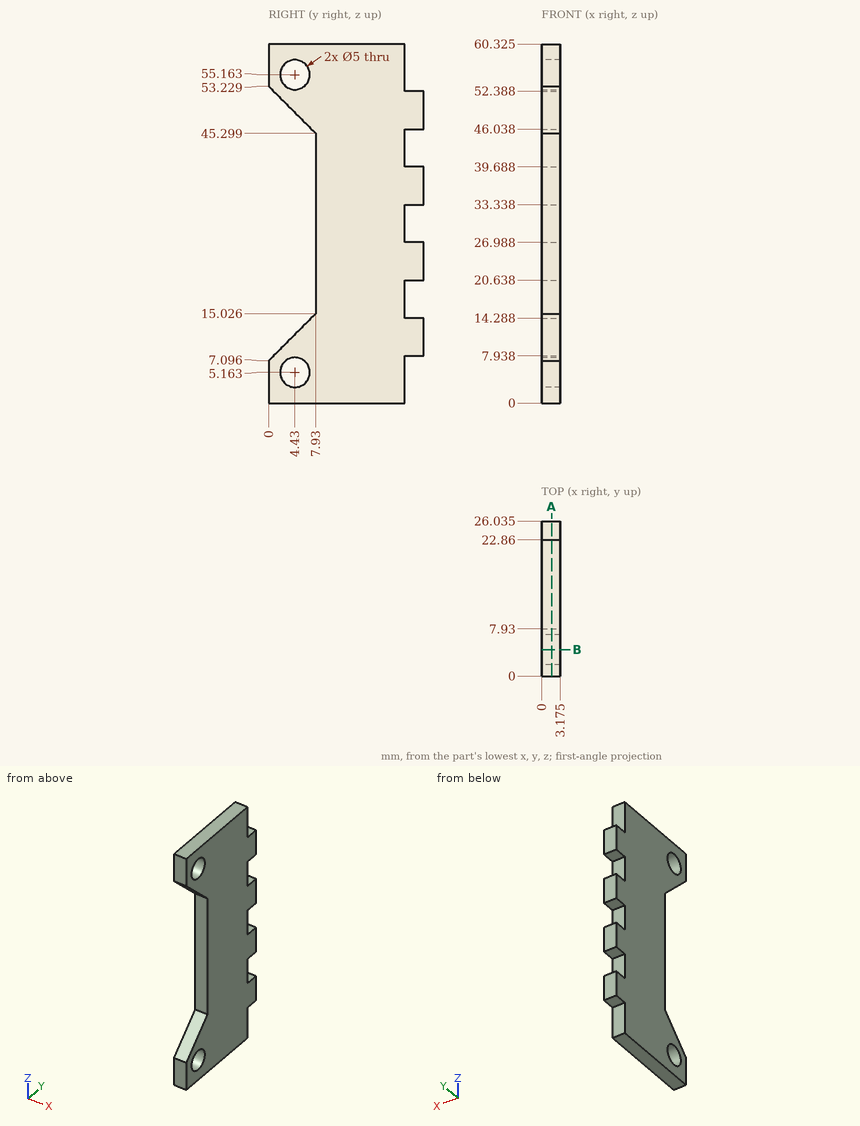
Study the drawing (mm; zero at the part's minimum x, y, z) and answer. Coordinates: 2 decimals unless noted, no trailing zeros. Write each loop counter-clockwise with the first axis right and the second up, starting at its lowest first coordinate (ties: lowest second). Pieces come first, ordered by that corner, then holes.
Q1. A cutting plane is placed at B-B, the plane y = 4.43. Give the vertices of the cut face in (x, z) (1 decimal).
Q2. Find the intervals of material crossed by line 1 (Z direction, x = 1.45, y = 24.25); line 2 (Z direction, x = 2.35, y = 6.5) (1 decimal); line 3 (Y direction, x = 2.05, z = 54.5), in increasing order.
Q3. A cutting plane is placed at A-A, the plane x = 1.7. Give the vertices of the cut face in (y, z) (1 decimal), then the cut area to 3 significant figures.
Q4. Each of these flat-tipped pins is pushed along its axis until it touches: pin 1 Ø1 at (x, z) = (1, 23) entering from -Y; pin 2 Ø1.6 at (x, z) = (1.5, 29) entering from +Y; pin 3 Ø1.6 at (x, y) = (2, 24) entering from -Z. Where does it stop, or does it pass through?
Findings below:
1. outline: (0, 0) - (3.2, 0) - (3.2, 2.7) - (0, 2.7) - close; (0, 7.7) - (3.2, 7.7) - (3.2, 11.5) - (0, 11.5) - close; (0, 48.8) - (3.2, 48.8) - (3.2, 52.7) - (0, 52.7) - close; (0, 57.7) - (3.2, 57.7) - (3.2, 60.3) - (0, 60.3) - close
2. line 1: z = 7.94 to 14.29, 20.64 to 26.99, 33.34 to 39.69, 46.04 to 52.39
2. line 2: z = 0 to 3.8, 6.6 to 13.6, 46.7 to 53.8, 56.6 to 60.3
2. line 3: y = 0 to 2.02, 6.84 to 22.86
3. outline: (0, 0) - (22.9, 0) - (22.9, 7.9) - (26, 7.9) - (26, 14.3) - (22.9, 14.3) - (22.9, 20.6) - (26, 20.6) - (26, 27) - (22.9, 27) - (22.9, 33.3) - (26, 33.3) - (26, 39.7) - (22.9, 39.7) - (22.9, 46) - (26, 46) - (26, 52.4) - (22.9, 52.4) - (22.9, 60.3) - (0, 60.3) - (0, 53.2) - (7.9, 45.3) - (7.9, 15) - (0, 7.1) - close; hole circle Ø5 at (4.4, 5.2); hole circle Ø5 at (4.4, 55.2)
3. area: 1,120 mm2
4. pin 1: stops at y = 7.93
4. pin 2: stops at y = 22.86
4. pin 3: stops at z = 7.94
